```python
from build123d import *

# Parameters (mm, degrees)
SKETCH2_R           = 10
BOSS_EXTRUDE5_DEPTH = 260
SKETCH5_W           = 12
SKETCH5_H           = 6
BOSS_EXTRUDE6_DEPTH = 40
SKETCH6_W           = 12
SKETCH6_H           = 6
BOSS_EXTRUDE7_DEPTH = 40


with BuildPart() as part:
    # Sketch2 → Boss-Extrude5 (new body)
    with BuildSketch(Plane.XY):
        Circle(SKETCH2_R)
    extrude(amount=BOSS_EXTRUDE5_DEPTH)

    # Sketch5 → Boss-Extrude6 (add)
    with BuildSketch(Plane.XY.offset(260)):
        with Locations((6, 0)):
            Rectangle(SKETCH5_W, SKETCH5_H)
    extrude(amount=-BOSS_EXTRUDE6_DEPTH)

    # Sketch6 → Boss-Extrude7 (add)
    with BuildSketch(Plane(origin=(0, 0, 0), x_dir=(-1, 0, 0), z_dir=(0, 0, -1))):
        with Locations((-6, 0)):
            Rectangle(SKETCH6_W, SKETCH6_H)
    extrude(amount=-BOSS_EXTRUDE7_DEPTH)


solid = part.part
```
Geometry check sheet. Reference: the model listing, model coordinates, mm. Coordinates: 2 decimals unless noted, no trailing zeros. Loops run counter-clockwise (first coordinate to the right, second up) from the corner with the lowest first, then second, coordinate; pieces in that order, holes last. Notation, with made-up numbers: (-30, 10) -> (-26, 10) arc R13 ccw to (-26, 31) -> close; hole circle Ø10 at (-26, 41). An arc over 180 degrees is marked (long way). Put each result on its own line as item: value.
1) Cross-section at A-A on y = 0. Record the boundary of the cut face in (x, z), plus the area to 3 significant figures.
Result set:
outline: (-10, 0) -> (12, 0) -> (12, 40) -> (10, 40) -> (10, 220) -> (12, 220) -> (12, 260) -> (-10, 260) -> close
area: 5,360 mm^2
2) Cross-section at D-D on z = 181.5. Record the boundary of the cut face in (x, y).
Result set:
outline: circle Ø20 at (0, 0)
3) Cross-section at B-B on z = 30. Record the boundary of the cut face in (x, y).
Result set:
outline: (9.54, -3) -> (12, -3) -> (12, 3) -> (9.54, 3) arc R10 ccw (long way) to start
4) Cross-section at C-C on x = -6.5. Record the boundary of the cut face in (y, z), plus the area to 3 significant figures.
Result set:
outline: (-7.6, 0) -> (7.6, 0) -> (7.6, 260) -> (-7.6, 260) -> close
area: 3,950 mm^2
5) Thickness scan on line 1 (Y direction, x = 11, z = 229); line 2 (X direction, y = 8.75, z = 219.5); line 3 (X direction, y = -6, z = 223.5). Record the ranges inside material, lowest first.
Result set:
line 1: y = -3 to 3
line 2: x = -4.84 to 4.84
line 3: x = -8 to 8
6) Gauge pin test, flat ends, axial feed: pin 1 Ø1.2 at (x, z) = (11.5, 29) entering from -Y; pin 2 Ø5 at (y, z) = (-7.5, 133) entering from -X; pin 3 Ø12 at (y, z) = (-7, 41.5) entering from -X. Record the tip position at first contact, or that the pin passes through.
Result set:
pin 1: stops at y = -3
pin 2: stops at x = -8.66
pin 3: stops at x = -9.95
